```python
from build123d import *

# Parameters (mm, degrees)
SKETCH2_W          = 1.5875
SKETCH2_H          = 13.97
CUT_EXTRUDE1_DEPTH = 3.175


with BuildPart() as part:
    # Sketch1 → Revolve1 (revolve)
    with BuildSketch(Plane.XY):
        Polygon((0, 4.7625), (0, 7.9375), (9.525, 7.9375), (9.525, 6.5405), (19.8374, 6.5405), (19.8374, 7.91718), (32.5374, 7.91718), (32.5374, 6.5405), (41.91, 6.5405), (49.53, 5.873836384), (49.53, 4.7625), align=None)
    revolve(axis=Axis((0, 0, 0), (1, 0, 0)))

    # Sketch2 → Cut-Extrude1 (cut)
    with BuildSketch(Plane.ZY):
        Rectangle(SKETCH2_W, SKETCH2_H)
    extrude(amount=-CUT_EXTRUDE1_DEPTH, mode=Mode.SUBTRACT)


solid = part.part
```
Read the model definition and answer for the solid it produces. Units are mm, in the model's axes. A direction names the side the tool comes from. Coordinates: 2 decimals unless noted, no trailing zeros. Write each loop counter-clockwise with the first axis right and the second up, starting at its lowest first coordinate (ties: lowest second). Pieces come first, ordered by that corner, then holes. Notation, with made-up numbers: (-33.5, -37.5) -> (-18.5, -37.5) arc R25 cw to (-18.5, -8.5) -> close; hole circle Ø9 at (67.25, 33). An arc over 180 degrees is marked (long way). Answer as a JSON object with one key per item and string values.
Q1. The part is cut by section C-C on x = 20.5. Give the vertices of the cut face in (y, z) (1 decimal).
The answers:
{"outline": "circle Ø15.8 at (0, 0); hole circle Ø9.5 at (0, 0)"}
Q2. The part is cut by section D-D on x = 35. Give the vertices of the cut face in (y, z) (1 decimal).
The answers:
{"outline": "circle Ø13.1 at (0, 0); hole circle Ø9.5 at (0, 0)"}
Q3. Determine the mould class of faces 1 (the flat face through (2, 6, 0.794)), 2 (the flat face through (0, 4, -3)), 3 (the conical face through (46.62, 3.29, 5.17)) for opening direction Z: pulls with the +Z half, pulls with the -Z half, needs draft (parallel to the pull), parting line crosses it, or undercut.
The answers:
{"face 1": "undercut", "face 2": "needs draft", "face 3": "parting line crosses it"}
Q4. The part is cut by section A-A on y = 0. Give the vertices of the cut face in (x, z) (1 decimal), then the cut area to 3 significant figures.
The answers:
{"outline": "(0, -7.9) -> (9.5, -7.9) -> (9.5, -6.5) -> (19.8, -6.5) -> (19.8, -7.9) -> (32.5, -7.9) -> (32.5, -6.5) -> (41.9, -6.5) -> (49.5, -5.9) -> (49.5, -4.8) -> (0, -4.8) -> close; (0, 4.8) -> (49.5, 4.8) -> (49.5, 5.9) -> (41.9, 6.5) -> (32.5, 6.5) -> (32.5, 7.9) -> (19.8, 7.9) -> (19.8, 6.5) -> (9.5, 6.5) -> (9.5, 7.9) -> (0, 7.9) -> close", "area": "233 mm2"}
Q5. The part is cut by section B-B on z = 0. Give the vertices of the cut face in (x, y) (1 decimal), then the cut area to 3 significant figures.
The answers:
{"outline": "(0, -7.9) -> (9.5, -7.9) -> (9.5, -6.5) -> (19.8, -6.5) -> (19.8, -7.9) -> (32.5, -7.9) -> (32.5, -6.5) -> (41.9, -6.5) -> (49.5, -5.9) -> (49.5, -4.8) -> (3.2, -4.8) -> (3.2, -7) -> (0, -7) -> close; (0, 7) -> (3.2, 7) -> (3.2, 4.8) -> (49.5, 4.8) -> (49.5, 5.9) -> (41.9, 6.5) -> (32.5, 6.5) -> (32.5, 7.9) -> (19.8, 7.9) -> (19.8, 6.5) -> (9.5, 6.5) -> (9.5, 7.9) -> (0, 7.9) -> close", "area": "219 mm2"}
Q6. Flat-ended cylindrical pins translate along their axes: pin 1 Ø5 at (x, z) = (43, 2.5) entering from +Y; pin 2 Ø5 at (x, y) = (18, -2) entering from +Z; pin 3 Ø3 at (x, y) = (20.5, -6) entering from +Z. Find the tip coordinate at first contact, or state that the pin passes through.
The answers:
{"pin 1": "stops at y = 6.54", "pin 2": "stops at z = 7.91", "pin 3": "stops at z = 6.51"}
Q7. Consider line 1 (Z direction, x = 25.5, y = 0); line 2 (X direction, y = 5.5, z = 4.5) (3 decimals); line 3 (Z direction, x = 11, y = 0). Determine where each line is inside the solid, lowest interval first. Write a range as [from, to].
The answers:
{"line 1": "z = [-7.92, -4.76], [4.76, 7.92]", "line 2": "x = [0, 9.525], [19.837, 32.537]", "line 3": "z = [-6.54, -4.76], [4.76, 6.54]"}
Q8. A tool of negligible diameter and unlimited length cuts with its end or side. For faces 4 (the flat face through (2, -6, -0.794)), 5 (the cylindrical face through (14.753, -0.851, 6.485)), 6 (the flat face through (32.537, -3, 6)), from which of +Z, -Z, +X, -X, +Y, -Y can it reach the whole face along a straight path? Write none if from no direction.
The answers:
{"face 4": "-X", "face 5": "none", "face 6": "+X"}
